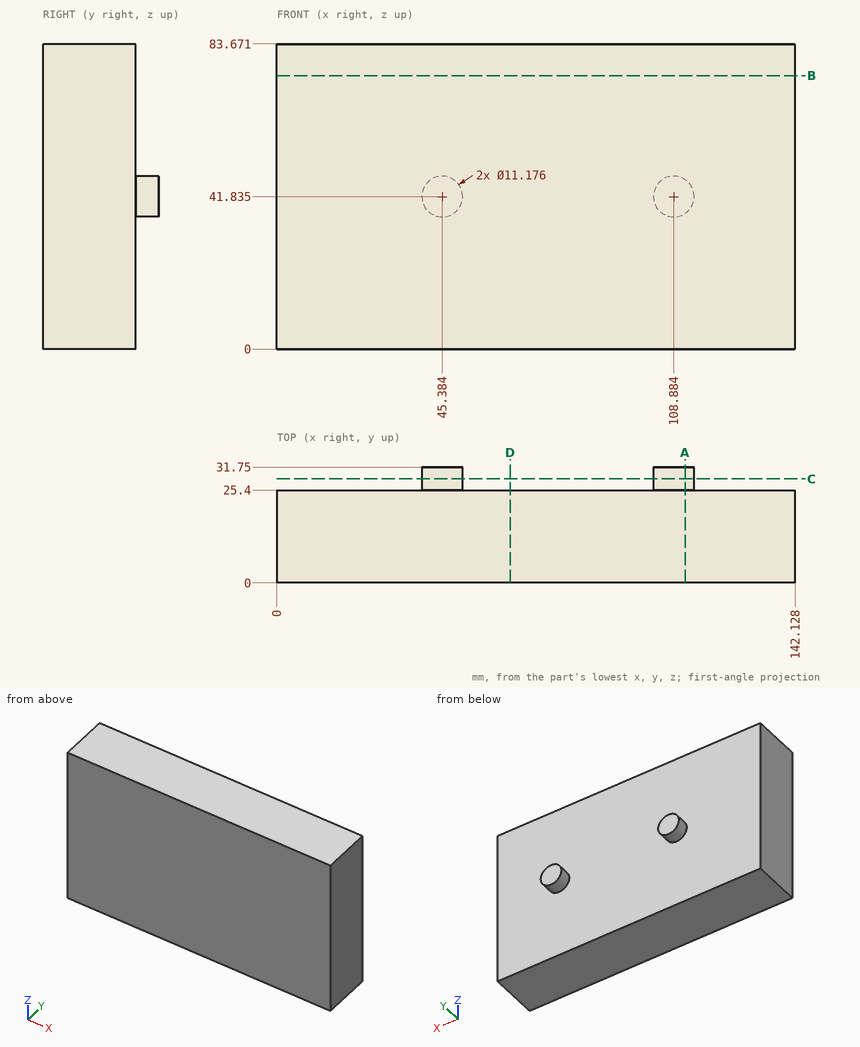
Part print with two shaded views. Sizes in mm from the minimum x, y, z corner. Coordinates: 2 decimals unless noted, no trailing zeros. Write each loop counter-clockwise with the first axis right and the second up, starting at its lowest first coordinate (ties: lowest second). Pieces come first, ordered by that corner, then holes.
(1) Cut at B-B on z = 75. List the corners of the cut face in (x, y), and give its area (3 significant figures).
(2) Pin check, flat tips, straight feed: pin 1 Ø10 at (y, z) = (10, 14) entering from -X; pin 2 Ø1 at (x, z) = (127.5, 44) entering from +Y. Stop position of each tip, or through.
(3) Cut at C-C on y = 28.5. List the corners of the cut face in (x, z) (1 decimal), and give its area (3 significant figures).
(4) Drill centre lines: line 1 (Y direction, x = 104.5, z = 79.5); line 2 (X direction, y = 27, z = 37) (1 decimal). Where is each one in solid material? Low to high.
(5) Cut at D-D on x = 64. List the corners of the cut face in (y, z).
(6) Cut at A-A on x = 112. List the corners of the cut face in (y, z).
Working result:
1. outline: (0, 0) - (142.13, 0) - (142.13, 25.4) - (0, 25.4) - close
1. area: 3,610 mm2
2. pin 1: stops at x = 0
2. pin 2: stops at y = 25.4
3. outline: circle Ø11.2 at (45.4, 41.8); circle Ø11.2 at (108.9, 41.8)
3. area: 196 mm2
4. line 1: y = 0 to 25.4
4. line 2: x = 42.6 to 48.2, 106.1 to 111.7
5. outline: (0, 0) - (25.4, 0) - (25.4, 83.67) - (0, 83.67) - close
6. outline: (0, 0) - (25.4, 0) - (25.4, 37.2) - (31.75, 37.2) - (31.75, 46.47) - (25.4, 46.47) - (25.4, 83.67) - (0, 83.67) - close
